Autodesk Inventor part; units mm, degrees
ref_plane "YZ Plane" through (0, 0, 0) normal (1, 0, 0) x (0, 1, 0)
ref_plane "XZ Plane" through (0, 0, 0) normal (0, 1, 0) x (-1, 0, 0)
ref_plane "XY Plane" through (0, 0, 0) normal (0, 0, 1) x (1, 0, 0)
sketch "Sketch1" plane through (0, 0, 0) normal (0, 1, 0) x (-1, 0, 0)
  line L0 (0, 0) -> (500, 0)
  arc A0 (500, 0) -> (399.5191, 375) centre (-250, 0) ccw
  arc A1 (0, 0) -> (-33.4936, 125) centre (-250, 0) ccw
  line L1 (-33.4936, 125) -> (399.5191, 375)
  line L2 (-404.937, 0) -> (679.6218, 0)
  dimension "d1" = 500
  dimension "d2" = 30
  dimension "d10" = 250
extrude "Extrusion1" add sketch "Sketch1" along normal blind 500
sketch "Sketch2" plane through (0, 500, 0) normal (0, 1, 0) x (1, 0, 0)
  arc A0 (0, 0) -> (33.4936, -125) centre (250, 0) ccw
  line L0 (33.4936, -125) -> (-399.5191, -375)
  arc A1 (-500, 0) -> (-399.5191, -375) centre (250, 0) ccw
  line L1 (-500, 0) -> (0, 0)
  line L2 (-387.9968, -333.7066) -> (-6.0913, -113.2133)
  arc A2 (-28.3882, -30) -> (-6.0913, -113.2133) centre (250, 0) ccw
  line L3 (-28.3882, -30) -> (-469.3747, -30)
  arc A3 (-469.3747, -30) -> (-387.9968, -333.7066) centre (250, 0) ccw
  dimension "d5" = 30
extrude "Extrusion2" cut sketch "Sketch2" against normal blind 200 contours A3 L3 A2 L2
fillet "Fillet2" radius 10 12 edges at (-183.0127, 500, 250) (8.5185, 0, 64.7048) (0, 250, 0) (8.5185, 500, 64.7048) (33.4936, 250, 125) (-474.4444, 0, 194.1143) (-399.5191, 250, 375) (-474.4444, 500, 194.1143) (-500, 250, 0) (-250, 0, 0) (-250, 500, 0) (-183.0127, 0, 250)
properties part number "angular30" material "Concrete"
Model file for the job. Use its own axes, mm. A direction names the side the tool comes from. Give positions to 0.01 mm unless a question says otherwise; leave off trailing zeros. Order: outer loops, then holes, each group sorted by start corner. A loop starts at its lowest first (then second) coordinate and runs counter-clockwise, first axis right, second up. Notation, with made-up numbers: M 10,18.5 L 36,18.5 A16 ccw 36,46.5 Z; hole C 1,-37 d11. An arc over 180 degrees is marked long. Write item = value, one per line.
Q1. Drill centre lines: line 1 (Y direction, x = -306.5, z = 122); line 2 (X direction, y = 307.5, z = 33); line 3 (X direction, y = 365.5, z = 126.5). Where is each one in solid material? Low to high. Write a range as [from, to].
Derived:
line_1 = [0, 300]
line_2 = [-499.27, -469.24], [-28.05, 2.19]
line_3 = [-489.25, -458.8], [-29.1, 28.51]
Q2. Tool access for faces 1 (the flat face through (-292, 300, 146)), 2 (the cylindrical face through (29.577, 253.36, 124.12)): list every direction of +Z, -Z, +X, -X, +Y, -Y with a clear straight run to the whole face (end or side of a thin tool).
Derived:
face_1 = +Y
face_2 = +X, +Y, -Y
Q3. Flat gauge pins, fed straight in: pin 1 (6 mm diameter, centred on y = 365, z = 204, fed in from -X); pin 2 (3 mm diameter, centred on y = 379.5, z = 300.5, fed in from +X); pin 3 (6 mm diameter, centred on y = 207, z = 320, fed in from -X). Where does each tip first touch, or does it go through?
Derived:
pin_1 = -472.56
pin_2 = -267.88
pin_3 = -429.71
Q4. Cut at A-A, the plane y = 334. List the corners of the cut face in (x, z), then the cut area to 3 significant figures.
Derived:
outline = M -499.93,10.14 A10 ccw -489.93,0 L -9.81,0 A10 ccw 0.18,9.62 A250 cw 28.85,116.58 A10 ccw 25,129.9 L -390.8,369.97 A10 ccw -404.53,366.19 A750 ccw Z; hole M -469.37,30 L -28.39,30 A280 cw -6.09,113.21 L -388,333.71 A720 ccw Z
area = 42,000 mm2
Q5. Two-plate mould, pull along X, no slides. Class faces 3 (the flat face through (-196, 500, 226)), 4 (the cylindrical face through (-187, 3, 249)), 5 (the cylindrical face through (-446.038, 401.4, 184.206)): pulls with the +X half, pulls with the -X half, needs draft (parallel to the pull), parting line crosses it, or undercut.
Derived:
face_3 = needs draft
face_4 = pulls with the +X half
face_5 = undercut
